The listing builds one solid part. Answer for the finished solid, in the listing's coordinates (mm). Give positions to 0.01 mm unless a question says otherwise; leave off trailing zeros. Write each loop counter-clockwise with the first axis right and the second up, starting at its lowest first coordinate (ties: lowest second). Pieces come first, ordered by that corner, then holes. Notation, with made-up numbers: (29.25, 51) - (58.25, 51) arc R23 ccw to (58.25, 72) - close; hole circle Ø6 at (82.5, 27.5). An arc over 180 degrees is marked (long way). One line per item, written item: value. Start each with the question number.
from build123d import *

# Parameters (mm, degrees)
SKETCH1_W           = 120
SKETCH1_H           = 180
BOSS_EXTRUDE1_DEPTH = 6
SKETCH2_R           = 5
CUT_EXTRUDE1_DEPTH  = 6
SKETCH4_R           = 22.5
SKETCH4_R_2         = 3
CUT_EXTRUDE3_DEPTH  = 10
SKETCH5_W           = 120
SKETCH5_H           = 7.698004818
CUT_EXTRUDE4_DEPTH  = 10
FILLET1_R           = 10


with BuildPart() as part:
    # Sketch1 → Boss-Extrude1 (new body)
    with BuildSketch(Plane(origin=(0, 0, 0), x_dir=(1, 0, 0), z_dir=(0, 1, 0))):
        Rectangle(SKETCH1_W, SKETCH1_H)
    extrude(amount=BOSS_EXTRUDE1_DEPTH)

    # Sketch2 → Cut-Extrude1 (cut)
    with BuildSketch(Plane(origin=(0, 6, 0), x_dir=(1, 0, 0), z_dir=(0, 1, 0))):
        with Locations(Location((-42.5, 75, 0), (0, 0, 270))):
            Circle(SKETCH2_R)
        with Locations(Location((42.5, 75, 0), (0, 0, 270))):
            Circle(SKETCH2_R)
        with Locations(Location((-42.5, -64, 0), (0, 0, 270))):
            Circle(SKETCH2_R)
        with Locations(Location((42.5, -64, 0), (0, 0, 270))):
            Circle(SKETCH2_R)
        with Locations(Location((0, 42.2, 0), (0, 0, 270))):
            Circle(SKETCH2_R)
    extrude(amount=-CUT_EXTRUDE1_DEPTH, mode=Mode.SUBTRACT)

    # Sketch4 → Cut-Extrude3 (cut)
    with BuildSketch(Plane(origin=(0, 6, 0), x_dir=(1, 0, 0), z_dir=(0, 1, 0))):
        with Locations(Location((0, -20.3, 0), (0, 0, 270))):
            Circle(SKETCH4_R)
        with Locations(Location((-28, -20.3, 0), (0, 0, 270))):
            Circle(SKETCH4_R_2)
        with Locations(Location((28, -20.3, 0), (0, 0, 270))):
            Circle(SKETCH4_R_2)
    extrude(amount=-CUT_EXTRUDE3_DEPTH, mode=Mode.SUBTRACT)

    # Sketch5 → Cut-Extrude4 (cut)
    with BuildSketch(Plane(origin=(0, 6, 0), x_dir=(1, 0, 0), z_dir=(0, 1, 0))):
        with Locations((0, -86.150997591)):
            Rectangle(SKETCH5_W, SKETCH5_H)
    extrude(amount=-CUT_EXTRUDE4_DEPTH, mode=Mode.SUBTRACT)

    # Fillet1
    fillet1_edges = [part.edges().sort_by_distance(p)[0] for p in [
        (-60, 3, 82.301995182),
        (60, 3, 82.301995182),
        (-60, 3, -90),
        (60, 3, -90),
    ]]
    fillet(fillet1_edges, radius=FILLET1_R)


solid = part.part
Item 1: Straight lines are drawn through the part: line 1 along X through (y, z) = (2.7, 64); line 2 along Z through (x, y) = (6.5, 5.2); line 3 along X through (y, z) = (2.5, 23). For each, find the intervals that lie inside material, in ascending order.
Item 2: The mould has two halves that part along X. Classify faces 1 (the cylindrical face through (47.457, 3.042, 63.349)), 2 (the flat face through (-60, 3, -3)), 3 (the cylindrical face through (56.993, 2.958, 79.45)): +X half, -X half, draft (parallel to the pull), parting line (faces both ways), or undercut.
Item 3: Find section A-A on x = 42.5. Determine the outline of the cut face in (y, z), plus the area to 3 significant figures.
Item 4: Find section B-B on z = 20.3. Determine the outline of the cut face in (x, y).
Item 5: Find section C-C on x = 18. Determine the outline of the cut face in (y, z).
Item 6: Find section D-D on z = -75. Determine the outline of the cut face in (x, y), plus the area to 3 significant figures.
Values:
1. line 1: -60 to -47.5, -37.5 to 37.5, 47.5 to 60
1. line 2: -90 to -1.24, 41.84 to 82.3
1. line 3: -60 to -29.31, -26.69 to -22.34, 22.34 to 26.69, 29.31 to 60
2. face 1: undercut
2. face 2: -X half
2. face 3: +X half
3. outline: (0, -90) - (6, -90) - (6, -80) - (0, -80) - close; (0, -70) - (6, -70) - (6, 59) - (0, 59) - close; (0, 69) - (6, 69) - (6, 82.3) - (0, 82.3) - close
3. area: 914 mm^2
4. outline: (-60, 0) - (-31, 0) - (-31, 6) - (-60, 6) - close; (-25, 0) - (-22.5, 0) - (-22.5, 6) - (-25, 6) - close; (22.5, 0) - (25, 0) - (25, 6) - (22.5, 6) - close; (31, 0) - (60, 0) - (60, 6) - (31, 6) - close
5. outline: (0, -90) - (6, -90) - (6, 6.8) - (0, 6.8) - close; (0, 33.8) - (6, 33.8) - (6, 82.3) - (0, 82.3) - close
6. outline: (-60, 0) - (-47.5, 0) - (-47.5, 6) - (-60, 6) - close; (-37.5, 0) - (37.5, 0) - (37.5, 6) - (-37.5, 6) - close; (47.5, 0) - (60, 0) - (60, 6) - (47.5, 6) - close
6. area: 600 mm^2
